Design review of the part built by this model. Coordinates are the model's own, in mm. Coordinates: 2 decimals unless noted, no trailing zeros. Loops run counter-clockwise (first coordinate to the right, second up) from the corner with the lowest first, then second, coordinate; pieces in that order, holes last. Notation, with made-up numbers: (-2.5, 88) - (38.5, 88) arc R13 ccw to (38.5, 103) - close; hole circle Ø9 at (-23, 84). An arc over 180 degrees is marked (long way). Use one line per item in the form item = value. Start each with the question number.
(1) Add section A-A (y = -7.5). State the section outline as (x, z) points.
(2) Add section B-B (y = 22.5). State the section outline as (x, z) points.
(3) Clearance check with flat-ended pins moving along their axes: pin 1 Ø1.8 at (x, y) = (-26.25, -7.5) entering from -Z; pin 2 Ø1.5 at (x, z) = (-33, -1.5) entering from +Y; pin 3 Ø2 at (y, z) = (-29.5, -1.5) entering from -X; pin 4 Ø1.8 at (x, y) = (-25.74, -10) entering from -Z. State where each tip first meets the part, or that it passes through.
(4) Add section D-D (x = -32). State the section outline as (y, z) points.
(5) Add section C-C (x = 21.5). State the section outline as (y, z) points, plus the area to 3 significant figures.
(6) For L1, parallel to X at y = -22.5, z = -3.5; L2, parallel to X at y = -23.5, z = -2.5; L3, parallel to Y at x = 21.5, z = -3.75, list the stretches that pass through material, from the lowest coordinate up.
Autodesk Inventor part; units mm, degrees
ref_plane "YZ Plane" through (0, 0, 0) normal (1, 0, 0) x (0, 1, 0)
ref_plane "XZ Plane" through (0, 0, 0) normal (0, 1, 0) x (-1, 0, 0)
ref_plane "XY Plane" through (0, 0, 0) normal (0, 0, 1) x (1, 0, 0)
sketch "Sketch1" plane through (0, 0, 0) normal (0, 0, 1) x (1, 0, 0)
  line L0 (35, 27.5) -> (-35, 27.5) construction
  line L1 (-35, 27.5) -> (-35, -27.5)
  line L2 (-35, -27.5) -> (35, -27.5) construction
  line L3 (35, -27.5) -> (35, 27.5)
  line L4 (35, 27.5) -> (-35, -27.5) construction
  line L5 (-35, 27.5) -> (35, -27.5) construction
  line L6 (0, 27.5) -> (0, -27.5) construction
  line L7 (35, 0) -> (-35, 0) construction
  line L8 (26, 27.5) -> (26, 30.5)
  line L9 (26, 30.5) -> (-26, 30.5)
  line L10 (-26, 30.5) -> (-26, 27.5)
  arc A0 (-29, 27.5) -> (-26, 27.5) centre (-27.5, 27.5) ccw
  line L11 (26, -27.5) -> (26, -30.5)
  line L12 (26, -30.5) -> (-26, -30.5)
  line L13 (-26, -30.5) -> (-26, -27.5)
  arc A1 (-26, -27.5) -> (-29, -27.5) centre (-27.5, -27.5) ccw
  line L14 (-32, 27.5) -> (-32, 21.5) construction
  line L15 (0, 30.5) -> (0, 27.5) construction
  line L16 (32, 27.5) -> (32, 21.5) construction
  arc A2 (26, 27.5) -> (29, 27.5) centre (27.5, 27.5) ccw
  arc A3 (29, -27.5) -> (26, -27.5) centre (27.5, -27.5) ccw
  line L17 (-17.5, -10) -> (-35, -10) construction
  line L18 (-35, -10) -> (-35, 10) construction
  line L19 (-35, 10) -> (-17.5, 10) construction
  line L20 (-17.5, 10) -> (-17.5, -10) construction
  line L21 (-17.5, -10) -> (-35, 10) construction
  line L22 (-35, -10) -> (-17.5, 10) construction
  line L23 (-26.25, -7.5) -> (-26.25, 7.5) construction
  line L24 (-25.7386, -10) -> (-25.7386, 10) construction
  circle A4 centre (-25.7386, 10) radius 2.5 construction
  line L25 (-33, 3.75) -> (-32, 3.75)
  line L26 (-30, 1.75) -> (-30, -1.75)
  line L27 (-32, -3.75) -> (-33, -3.75)
  arc A5 (-32, -3.75) -> (-30, -1.75) centre (-32, -1.75) ccw
  arc A6 (-30, 1.75) -> (-32, 3.75) centre (-32, 1.75) ccw
  arc A7 (-35, 5.75) -> (-33, 3.75) centre (-33, 5.75) ccw
  line L28 (35, -27.5) -> (29, -27.5)
  line L29 (-29, -27.5) -> (-35, -27.5)
  line L30 (-35, 27.5) -> (-29, 27.5)
  line L31 (29, 27.5) -> (35, 27.5)
  circle A8 centre (-26.25, 7.5) radius 2.5 construction
  line L32 (14.2614, -25) -> (-20.7386, -25) construction
  line L33 (-20.7386, -25) -> (-20.7386, 25) construction
  line L34 (-20.7386, 25) -> (14.2614, 25) construction
  line L35 (14.2614, 25) -> (14.2614, -25) construction
  line L36 (14.2614, -25) -> (-20.7386, 25) construction
  line L37 (-20.7386, -25) -> (14.2614, 25) construction
  line L38 (11.7614, 22.5) -> (-18.2386, 22.5) construction
  line L39 (-18.2386, 22.5) -> (-18.2386, -22.5) construction
  line L40 (-18.2386, -22.5) -> (11.7614, -22.5) construction
  line L41 (11.7614, -22.5) -> (11.7614, 22.5) construction
  line L42 (11.7614, 22.5) -> (-18.2386, -22.5) construction
  line L43 (-18.2386, 22.5) -> (11.7614, -22.5) construction
  circle A9 centre (-18.2386, 22.5) radius 2.5 construction
  arc A10 (-21.2236, 22.2) -> (-15.2536, 22.2) centre (-18.2386, 22.5) ccw
  line L44 (-21.2386, 10) -> (-21.2386, 3)
  line L45 (-13.2637, 24) -> (6.7865, 24)
  arc A11 (8.7764, 22.2) -> (14.7464, 22.2) centre (11.7614, 22.5) ccw
  arc A12 (32.802, 10.6698) -> (32.3609, 9.408) centre (46.2004, 5.2778) ccw
  line L46 (32.9466, 11.4165) -> (32.9466, 22)
  line L47 (30.9466, 24) -> (16.7363, 24)
  arc A13 (32.802, 10.6698) -> (32.9466, 11.4165) centre (30.9466, 11.4165) ccw
  line L48 (34.9466, 11.4165) -> (32.9466, 11.4165) construction
  line L49 (32.802, 8.6698) -> (32.802, 10.6698) construction
  line L50 (30.4444, 7.9799) -> (22.1342, 7.9799)
  line L51 (15.9549, 1.8007) -> (15.9549, 3)
  line L52 (13.9549, 1) -> (-19.2386, 1)
  arc A14 (30.4444, 7.9799) -> (32.3609, 9.408) centre (30.4444, 9.9799) ccw
  arc A15 (32.9466, 22) -> (30.9466, 24) centre (30.9466, 22) ccw
  arc A16 (16.7363, 24) -> (14.7464, 22.2) centre (16.7363, 22) ccw
  arc A17 (8.7764, 22.2) -> (6.7865, 24) centre (6.7865, 22) ccw
  arc A18 (-13.2637, 24) -> (-15.2536, 22.2) centre (-13.2637, 22) ccw
  arc A19 (-21.2386, 3) -> (-19.2386, 1) centre (-19.2386, 3) ccw
  arc A20 (13.9549, 1) -> (15.9549, 3) centre (13.9549, 3) ccw
  arc A21 (22.1342, 7.9799) -> (15.9549, 1.8007) centre (22.1342, 1.8007) ccw
  arc A22 (-15.2536, -22.2) -> (-21.2236, -22.2) centre (-18.2386, -22.5) ccw
  line L53 (-21.2386, -10) -> (-21.2386, -3)
  line L54 (-13.2637, -24) -> (6.7865, -24)
  arc A23 (14.7464, -22.2) -> (8.7764, -22.2) centre (11.7614, -22.5) ccw
  arc A24 (32.3609, -9.408) -> (32.802, -10.6698) centre (46.2004, -5.2778) ccw
  line L55 (32.9466, -11.4165) -> (32.9466, -22)
  line L56 (30.9466, -24) -> (16.7363, -24)
  arc A25 (32.9466, -11.4165) -> (32.802, -10.6698) centre (30.9466, -11.4165) ccw
  line L57 (30.4444, -7.9799) -> (22.1342, -7.9799)
  line L58 (15.9549, -1.8007) -> (15.9549, -3)
  line L59 (13.9549, -1) -> (-19.2386, -1)
  arc A26 (32.3609, -9.408) -> (30.4444, -7.9799) centre (30.4444, -9.9799) ccw
  arc A27 (30.9466, -24) -> (32.9466, -22) centre (30.9466, -22) ccw
  arc A28 (14.7464, -22.2) -> (16.7363, -24) centre (16.7363, -22) ccw
  arc A29 (6.7865, -24) -> (8.7764, -22.2) centre (6.7865, -22) ccw
  arc A30 (-15.2536, -22.2) -> (-13.2637, -24) centre (-13.2637, -22) ccw
  arc A31 (-19.2386, -1) -> (-21.2386, -3) centre (-19.2386, -3) ccw
  arc A32 (15.9549, -3) -> (13.9549, -1) centre (13.9549, -3) ccw
  arc A33 (15.9549, -1.8007) -> (22.1342, -7.9799) centre (22.1342, -1.8007) ccw
  line L60 (-32.9466, 13.8893) -> (-32.9466, 22)
  arc A34 (-30.9466, 24) -> (-32.9466, 22) centre (-30.9466, 22) ccw
  arc A35 (-21.2236, 22.2) -> (-23.2135, 24) centre (-23.2135, 22) ccw
  line L61 (-30.9466, 24) -> (-23.2135, 24)
  arc A36 (-21.2386, 10) -> (-29.3442, 12.6926) centre (-25.7386, 10) ccw
  arc A37 (-32.9466, 13.8893) -> (-29.3442, 12.6926) centre (-30.9466, 13.8893) ccw
  line L62 (-32.9466, -13.8893) -> (-32.9466, -22)
  arc A38 (-32.9466, -22) -> (-30.9466, -24) centre (-30.9466, -22) ccw
  line L63 (-30.9466, -24) -> (-23.2135, -24)
  arc A39 (-29.3442, -12.6926) -> (-21.2386, -10) centre (-25.7386, -10) ccw
  arc A40 (-29.3442, -12.6926) -> (-32.9466, -13.8893) centre (-30.9466, -13.8893) ccw
  arc A41 (-23.2135, -24) -> (-21.2236, -22.2) centre (-23.2135, -22) ccw
  line L64 (25, -16) -> (-25, -16) construction
  line L65 (-25, -16) -> (-25, 16) construction
  line L66 (-25, 16) -> (25, 16) construction
  line L67 (25, 16) -> (25, -16) construction
  line L68 (25, -16) -> (-25, 16) construction
  line L69 (-25, -16) -> (25, 16) construction
  line L70 (21.5, -12.5) -> (21.5, 12.5) construction
  point P0 (0, 0)
  point P1 (0, 0)
  point P2 (0, -0.0008)
  point P3 (-29, -27.5)
  point P4 (26, -27.5)
  point P5 (-26, -27.5)
  point P6 (-26, -27.5)
  point P7 (26, -27.5)
  point P8 (-26.25, 0)
  point P9 (29, -27.5)
  point P10 (29, -10)
  point P11 (-3.2386, 0)
  point P12 (-21.2386, 22.5)
  point P13 (-15.6405, 24)
  point P14 (9.1633, 24)
  point P15 (14.3595, 24)
  point P16 (32.0128, 7.9799)
  point P17 (0, 0)
  dimension "d19" = 3
  dimension "d20" = 52
  dimension "d37" = 55
  dimension "d40" = 6
  dimension "d41" = 6
  dimension "d59" = 70
  dimension "d60" = 1.5
  dimension "d61" = 17.5
  dimension "d62" = 20
  dimension "d63" = 15
  dimension "d90" = 20
  dimension "d98" = 5
  dimension "d100" = 7.5
  dimension "d101" = 5
  dimension "d111" = 5
  dimension "d113" = 50
  dimension "d114" = 35
  dimension "d115" = 5
  dimension "d117" = 5
  dimension "d118" = 2
  dimension "d119" = 2
  dimension "d120" = 2
  dimension "d124" = 2
  dimension "d125" = 2
  dimension "d126" = 3
  dimension "d128" = 50
  dimension "d129" = 32
  dimension "d130" = 25
  dimension "d131" = 3.5
  dimension "d140" = 0
  dimension "d141" = 10
extrude "Extrusion1" add sketch "Sketch1" against normal blind 5 contours L30 A0 L10 L9 L8 A2 L31 L3 L28 A3 L11 L12 L13 A1 L29 L1 | A10 A18 L45 A17 A11 A16 L47 A15 L46 A13 A12 A14 L50 A21 L51 A20 L52 A19 L44 A36 A37 L60 A34 L61 A35 | A22 A41 L63 A38 L62 A40 A39 L53 A31 L59 A32 L58 A33 L57 A26 A24 A25 L55 A27 L56 A28 A23 A29 L54 A30
hole "M2" at (-26.25, -7.5, 0) at (-26.25, 7.5, 0) at (11.7614, 22.5, 0) at (-18.2386, 22.5, 0) at (-18.2386, -22.5, 0) at (11.7614, -22.5, 0) direction (0, 0, -1) diameter 1.567 end through all
hole "Phi3" at (-25.7386, -10, 0) at (-25.7386, 10, 0) direction (0, 0, -1) diameter 3 end through all
sketch "Sketch3" plane through (29, 27.5, 0) normal (0, 1, 0) x (1, 0, 0)
  line L0 (6, 0) -> (0, 0)
  line L1 (3, 0) -> (3, 5)
  line L2 (-58, 0) -> (-64, 0)
  line L3 (-61, 0) -> (-61, 5)
  line L4 (-64, 5) -> (-58, 5)
  line L5 (0, 5) -> (6, 5)
  point P0 (-29, 0)
  point P1 (3, 0)
  point P2 (3, 2.5)
  point P3 (-61, 2.5)
hole "Side-M2" at (32, 27.5, -2.5) at (-32, 27.5, -2.5) direction (0, -1, 0) diameter 1.567 depth 6.3
chamfer "C0.5" distance 0.5 angle 45 4 edges at (26, -30.5, -2.5) (-26, -30.5, -2.5) (26, 30.5, -2.5) (-26, 30.5, -2.5)
mirror "Mirror1" about plane through (0, 0, 0) normal (0, 1, 0) of "Side-M2"
hole "Hole6" at (21.5, -12.5, 0) at (21.5, 12.5, 0) direction (0, 0, -1) diameter 2.459 end through all
properties part number "HeadCircuitMountFrame" material "Acetal Resin, Black"
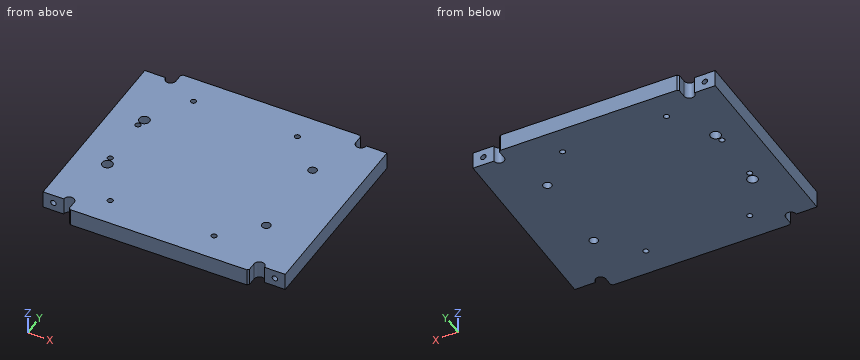
Computed values:
q1.outline = (-35, -5) - (-27.03, -5) - (-27.03, 0) - (-35, 0) - close; (-25.47, -5) - (35, -5) - (35, 0) - (-25.47, 0) - close
q2.outline = (-35, -5) - (-19.02, -5) - (-19.02, 0) - (-35, 0) - close; (-17.46, -5) - (10.98, -5) - (10.98, 0) - (-17.46, 0) - close; (12.54, -5) - (35, -5) - (35, 0) - (12.54, 0) - close; hole circle Ø1.57 at (-32, -2.5); hole circle Ø1.57 at (32, -2.5)
q3.pin_1 = -5
q3.pin_2 = 27.5
q3.pin_3 = -26
q3.pin_4 = through
q4.outline = (-27.5, -5) - (27.5, -5) - (27.5, -3.28) - (21.2, -3.28) - (21.2, -1.72) - (27.5, -1.72) - (27.5, 0) - (-27.5, 0) - (-27.5, -1.72) - (-21.2, -1.72) - (-21.2, -3.28) - (-27.5, -3.28) - close
q5.outline = (-30.5, -5) - (-13.73, -5) - (-13.73, 0) - (-30.5, 0) - close; (-11.27, -5) - (11.27, -5) - (11.27, 0) - (-11.27, 0) - close; (13.73, -5) - (30.5, -5) - (30.5, 0) - (13.73, 0) - close
q5.area = 280 mm^2
q6.L1 = -35 to -19.02, -17.46 to 10.98, 12.54 to 35
q6.L2 = -35 to -32.78, -31.22 to 31.22, 32.78 to 35
q6.L3 = -30.5 to -13.73, -11.27 to 11.27, 13.73 to 30.5
